Autodesk Inventor part; units mm, degrees
ref_plane "Work Plane2" through (40.2, -14.35, 43.3) normal (0, 0, 1) x (1, 0, 0)
ref_plane "YZ Plane" through (0, 0, 0) normal (1, 0, 0) x (0, 1, 0)
ref_plane "XZ Plane" through (0, 0, 0) normal (0, 1, 0) x (-1, 0, 0)
ref_plane "Work Plane1" through (0, 0, 0) normal (0, 0, 1) x (1, 0, 0)
ref_plane "Work Plane2" through (40.2, -14.35, 43.3) normal (0, 0, 1) x (1, 0, 0)
sketch "Sketch1" plane through (0, 0, 0) normal (0, 0, 1) x (1, 0, 0)
  circle A0 centre (31.8, -10.75) radius 1.4
  circle A1 centre (63.8, -10.75) radius 1.4
  circle A2 centre (63.8, -2.75) radius 1.4
  circle A3 centre (31.8, -2.75) radius 1.4
  circle A4 centre (47.8, -6.75) radius 3.0846
  line L0 (21, -14.5) -> (21, 1)
  line L1 (21, -14.5) -> (74.6, -14.5)
  line L2 (74.6, 1) -> (74.6, -14.5)
  line L3 (21, 1) -> (74.6, 1)
  circle A5 centre (47.8, -6.75) radius 2.196 construction
  line L4 (55.4, 0.85) -> (40.2, 0.85) construction
  line L5 (40.2, 0.85) -> (40.2, -14.35) construction
  line L6 (40.2, -14.35) -> (55.4, -14.35) construction
  line L7 (55.4, -14.35) -> (55.4, 0.85) construction
  line L8 (68.8, -14.5) -> (58.8, -14.5)
  line L9 (58.8, -14.5) -> (58.8, 1)
  line L10 (58.8, 1) -> (68.8, 1)
  line L11 (68.8, 1) -> (68.8, -14.5)
  line L12 (68.8, -14.5) -> (58.8, 1) construction
  line L13 (58.8, -14.5) -> (68.8, 1) construction
  line L14 (36.8, -14.5) -> (26.8, -14.5)
  line L15 (26.8, -14.5) -> (26.8, 1)
  line L16 (26.8, 1) -> (36.8, 1)
  line L17 (36.8, 1) -> (36.8, -14.5)
  line L18 (36.8, -14.5) -> (26.8, 1) construction
  line L19 (26.8, -14.5) -> (36.8, 1) construction
  line L20 (26.8, -14.5) -> (68.8, -14.5)
  line L21 (68.8, -14.5) -> (68.8, -18.5)
  line L22 (68.8, -18.5) -> (26.8, -18.5)
  line L23 (26.8, -18.5) -> (26.8, -14.5)
  point P0 (0, 0)
  point P1 (63.8, -6.75)
  point P2 (31.8, -6.75)
  dimension "d0" = 10
  dimension "d1" = 15.5
  dimension "d2" = 0
  dimension "d3" = 10
  dimension "d4" = 15.5
  dimension "d7" = 4
extrude "Extrusion1" add sketch "Sketch1" along normal up to surface (43.3 mm away) contours L15 L3 L17 L1 | L1 L21 L22 L23 | L9 L3 L11 L1
sketch "Sketch2" plane through (26.8, -18.5, 0) normal (0, -1, 0) x (1, 0, 0)
  circle A0 centre (20.9, 34.8462) radius 1
  circle A1 centre (20.9, 19.8462) radius 1
  line L0 (13.4, 13) -> (28.6, 13)
  line L1 (28.6, 13) -> (28.6, 43.3)
  line L2 (13.4, 43.3) -> (28.6, 43.3)
  line L3 (13.4, 13) -> (13.4, 43.3)
  point P0 (-26.8, 0)
hole "Hole1" at (47.7, -18.5, 19.8462) at (47.7, -18.5, 34.8462) direction (0, 1, 0) diameter 3.2 end through all
chamfer "Chamfer1" distance 4 angle 45 2 edges at (26.8, -18.5, 21.65) (68.8, -18.5, 21.65)
sketch "Sketch3" plane through (36.8, -14.5, 43.3) normal (0, 0, 1) x (1, 0, 0)
  line L0 (32, 0) -> (28, -4)
  line L1 (32, 15.5) -> (32, 0)
  line L2 (22, 15.5) -> (32, 15.5)
  line L3 (22, 0) -> (22, 15.5)
  line L4 (0, 0) -> (22, 0)
  line L5 (0, 15.5) -> (0, 0)
  line L6 (-10, 15.5) -> (0, 15.5)
  line L7 (-10, 0) -> (-10, 15.5)
  line L8 (-6, -4) -> (-10, 0)
  line L9 (28, -4) -> (-6, -4)
  circle A0 centre (27, 3.75) radius 1.4
  circle A1 centre (27, 11.75) radius 1.4
  circle A2 centre (-5, 3.75) radius 1.4
  circle A3 centre (-5, 11.75) radius 1.4
  line L10 (-10, 0) -> (32, 0)
  point P0 (-36.8, 14.5)
extrude "Extrusion2" cut sketch "Sketch3" against normal blind 35 contours L10 L3 L2 L1 | L10 L7 L6 L5
fillet "Fillet1" radius 5 2 edges at (63.8, -14.5, 8.3) (31.8, -14.5, 8.3)
properties part number "31_MTP_wellplate_Solenoid_adapter"
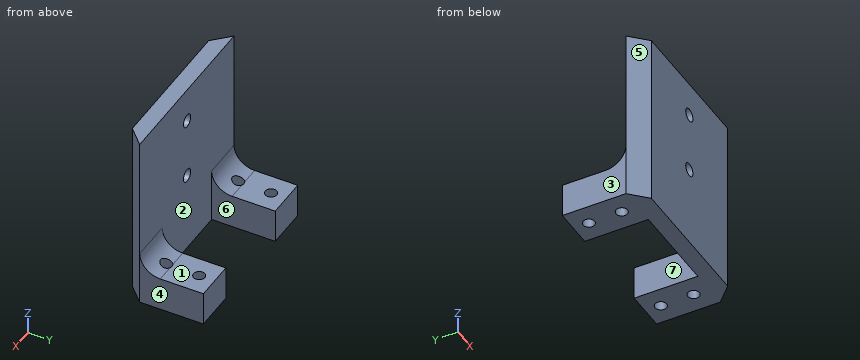
Build history of the part. All positions in model axes, mm. Face numbers are marked on the shaded views. A direction names the side the tool comes from. Coordinates: 2 decimals unless noted, no trailing zeros. Write each loop counter-clockwise with the first axis right and the second up, starting at its lowest first coordinate (ties: lowest second). Pieces come first, ordered by that corner, then holes. Notation, with made-up numbers: (18, 24) -> (32, 24) arc R21 ccw to (32, 55) -> close; hole circle Ø9 at (69, 59). An arc over 180 degrees is marked (long way). Use CSV: the item, a comma, the result in double quotes. Start each with the question number.
Q1. Cut at C-C, the plane y = -2.75. List the corners of the cut face in (x, z).
Q2. Drill centre lines: probe 1 along Y at (x, z) = (31.8, 2); probe 2 along Z at (x, y) = (47.7, -15.25); probe 3 along X at (y, z) = (-11.25, 6.5). Where is each one in solid material? Low to high.
Q3. Cut at A-A, the plane y = -8.25. List the corners of the cut face in (x, z).
Q4. Pull direction X, two halves, no side cores. Call the marked faces 4, 5, 6 and 7: released by +X, released by -X, zero draft, split by the parting line, or undercut.
Q5. Cut at D-D, the plane z = 19. List the corners of the cut face in (x, y).
Q6. Cut at B-B, the plane x = 31.8. List the corners of the cut face in (y, z).
Q7. Flat gauge pins, fed straight in: pin 1 Ø8 at (x, y) = (38.5, -8) entering from +Z; pin 2 Ø1.5 at (y, z) = (-16, 31) entering from +X; pin 3 Ø1.9 at (x, z) = (47.7, 19.85) entering from +Y (1 decimal); pin 4 Ø8 at (x, y) = (34, -7) entering from +Z. Where does each tip first touch, or does it go through?
Q8. 3-axis set-ups, long thin cutter, end or side, ignore diameter. For the marked faces 1, 2 and 3: which of +Z, -Z, +X, -X, +Y, -Y reach the whole face in a straight line?
Checked values:
1,outline,"(26.8, 0) -> (30.4, 0) -> (30.4, 8.3) -> (26.8, 8.3) -> close; (33.2, 0) -> (36.8, 0) -> (36.8, 8.3) -> (33.2, 8.3) -> close; (58.8, 0) -> (62.4, 0) -> (62.4, 8.3) -> (58.8, 8.3) -> close; (65.2, 0) -> (68.8, 0) -> (68.8, 8.3) -> (65.2, 8.3) -> close"
2,probe 1,"y = -18.5 to -12.15, -9.35 to -4.15, -1.35 to 1"
2,probe 2,"z = 0 to 18.25, 21.45 to 33.25, 36.45 to 43.3"
2,probe 3,"x = 26.8 to 30.49, 33.11 to 36.8, 58.8 to 62.49, 65.11 to 68.8"
3,outline,"(26.8, 0) -> (36.8, 0) -> (36.8, 8.3) -> (26.8, 8.3) -> close; (58.8, 0) -> (68.8, 0) -> (68.8, 8.3) -> (58.8, 8.3) -> close"
4,face 4,"released by +X"
4,face 5,"released by -X"
4,face 6,"undercut"
4,face 7,"undercut"
5,outline,"(26.8, -14.5) -> (30.8, -18.5) -> (46.34, -18.5) -> (46.34, -14.5) -> close; (49.06, -18.5) -> (64.8, -18.5) -> (68.8, -14.5) -> (49.06, -14.5) -> close"
6,outline,"(-18.5, 0) -> (-12.15, 0) -> (-12.15, 9.06) arc R5 cw to (-14.5, 13.3) -> (-14.5, 43.3) -> (-18.5, 43.3) -> close; (-9.35, 0) -> (-4.15, 0) -> (-4.15, 8.3) -> (-9.35, 8.3) -> close; (-1.35, 0) -> (1, 0) -> (1, 8.3) -> (-1.35, 8.3) -> close"
7,pin 1,"stops at z = 8.77"
7,pin 2,"stops at x = 68.05"
7,pin 3,"passes through"
7,pin 4,"stops at z = 8.53"
8,face 1,"+Z, +X, -X, +Y"
8,face 2,"+Z, +Y"
8,face 3,"+Z, -Z, -X, +Y, -Y"
